Model file for the job. Use its own axes, mm. A direction names the side the tool comes from. Round coordinates to 2 decimals unless told otherwise and drop trailing zeros. Loops run counter-clockwise (first coordinate to the right, second up) from the corner with the lowest first, then second, coordinate; pieces in that order, holes last. Notation, with made-up numbers: (48.5, 26) - (93.5, 26) arc R27 cw to (93.5, 51) - close; hole circle Ø6 at (86, -24.5). An arc over 180 degrees is marked (long way). Use one line per item in the form item = value.
from build123d import *

# Parameters (mm, degrees)
SKETCH2_W           = 60
SKETCH2_H           = 110
BOSS_EXTRUDE1_DEPTH = 1.5748
BOSS_EXTRUDE2_DEPTH = 6
BOSS_EXTRUDE3_DEPTH = 6
SKETCH6_W           = 6
SKETCH6_H           = 12.6
SKETCH6_W_2         = 7.6
SKETCH6_H_2         = 9.9
SKETCH6_W_3         = 3
SKETCH6_H_3         = 4.5
SKETCH6_W_4         = 16.25
SKETCH6_H_4         = 13.5
SKETCH6_W_5         = 3.65
SKETCH6_H_5         = 4.8
BOSS_EXTRUDE4_DEPTH = 1
SKETCH7_R           = 1.375
SKETCH7_R_2         = 1.625
CUT_EXTRUDE1_DEPTH  = 126.443214245
SKETCH8_R           = 0.9
BOSS_EXTRUDE5_DEPTH = 1
SKETCH9_W           = 2.7
SKETCH9_H           = 1.5
BOSS_EXTRUDE6_DEPTH = 1
CUT_EXTRUDE2_DEPTH  = 3


with BuildPart() as part:
    # Sketch2 → Boss-Extrude1 (new body)
    with BuildSketch(Plane(origin=(0, 0, 0), x_dir=(1, 0, 0), z_dir=(0, 1, 0))):
        with Locations((30, 55)):
            Rectangle(SKETCH2_W, SKETCH2_H)
    extrude(amount=-BOSS_EXTRUDE1_DEPTH)

    # Sketch3 → Boss-Extrude2 (add)
    with BuildSketch(Plane(origin=(0, 0, 0), x_dir=(1, 0, 0), z_dir=(0, 1, 0))):
        Polygon((0.6425, 8.49), (6.3575, 8.49), (6.3575, 21.5075), (7.31, 21.5075), (7.31, 28.4925), (6.3575, 28.4925), (6.3575, 41.51), (0.6425, 41.51), align=None)
    extrude(amount=BOSS_EXTRUDE2_DEPTH)

    # Sketch5 → Boss-Extrude3 (add)
    with BuildSketch(Plane(origin=(0, 0, 0), x_dir=(1, 0, 0), z_dir=(0, 1, 0))):
        Polygon((49.05, 109.3575), (10.95, 109.3575), (10.95, 103.6425), (26.5075, 103.6425), (26.5075, 102.69), (33.4925, 102.69), (33.4925, 103.6425), (49.05, 103.6425), align=None)
    extrude(amount=BOSS_EXTRUDE3_DEPTH)

    # Sketch6 → Boss-Extrude4 (add)
    with BuildSketch(Plane(origin=(0, 0, 0), x_dir=(1, 0, 0), z_dir=(0, 1, 0))):
        with Locations((33, 67)):
            Rectangle(SKETCH6_W, SKETCH6_H)
        Polygon((30.875, 33.85), (30.875, 27.65), (30.6, 27.375), (24.4, 27.375), (24.125, 27.65), (24.125, 33.85), (24.4, 34.125), (30.6, 34.125), align=None)
        with Locations((18.25, 13)):
            Rectangle(SKETCH6_W_2, SKETCH6_H_2)
        with Locations((23.5, 3.25)):
            Rectangle(SKETCH6_W_3, SKETCH6_H_3)
        with Locations((50.625, 17.25)):
            Rectangle(SKETCH6_W_4, SKETCH6_H_4)
        with Locations((57.75, 38)):
            Rectangle(SKETCH6_W_5, SKETCH6_H_5)
        with Locations((57.75, 45.25)):
            Rectangle(SKETCH6_W_5, SKETCH6_H_5)
        with Locations((51, 45)):
            Rectangle(SKETCH6_W_5, SKETCH6_H_5)
        with Locations((51, 35.5)):
            Rectangle(SKETCH6_W_5, SKETCH6_H_5)
    extrude(amount=BOSS_EXTRUDE4_DEPTH)

    # Sketch7 → Cut-Extrude1 (cut, through all)
    with BuildSketch(Plane(origin=(0, 0, 0), x_dir=(1, 0, 0), z_dir=(0, 1, 0))):
        with Locations(Location((3.75, 52, 0), (0, 0, 270))):
            Circle(SKETCH7_R)
        with Locations(Location((3.75, 70.5, 0), (0, 0, 270))):
            Circle(SKETCH7_R)
        with Locations(Location((3.75, 79.5, 0), (0, 0, 270))):
            Circle(SKETCH7_R)
        with Locations(Location((3.75, 88.5, 0), (0, 0, 270))):
            Circle(SKETCH7_R)
        with Locations(Location((3.75, 97.5, 0), (0, 0, 270))):
            Circle(SKETCH7_R)
        with Locations(Location((3.75, 61, 0), (0, 0, 270))):
            Circle(SKETCH7_R)
        with Locations(Location((5, 106, 0), (0, 0, 270))):
            Circle(SKETCH7_R_2)
        with Locations(Location((55, 106, 0), (0, 0, 270))):
            Circle(SKETCH7_R_2)
        with Locations(Location((55, 4, 0), (0, 0, 270))):
            Circle(SKETCH7_R_2)
        with Locations(Location((5, 4, 0), (0, 0, 270))):
            Circle(SKETCH7_R_2)
    extrude(amount=-CUT_EXTRUDE1_DEPTH, mode=Mode.SUBTRACT)

    # Sketch8 → Boss-Extrude5 (add)
    with BuildSketch(Plane(origin=(0, 1, 0), x_dir=(1, 0, 0), z_dir=(0, 1, 0))):
        with Locations(Location((57.75, 38, 0), (0, 0, 270))):
            Circle(SKETCH8_R)
        with Locations(Location((57.75, 45.25, 0), (0, 0, 270))):
            Circle(SKETCH8_R)
        with Locations(Location((51, 45, 0), (0, 0, 270))):
            Circle(SKETCH8_R)
        with Locations(Location((51, 35.5, 0), (0, 0, 270))):
            Circle(SKETCH8_R)
    extrude(amount=BOSS_EXTRUDE5_DEPTH)

    # Sketch9 → Boss-Extrude6 (add)
    with BuildSketch(Plane(origin=(0, 0, 0), x_dir=(1, 0, 0), z_dir=(0, 1, 0))):
        with Locations((57.5, 50)):
            Rectangle(SKETCH9_W, SKETCH9_H)
        with Locations((57.5, 54.25)):
            Rectangle(SKETCH9_W, SKETCH9_H)
        with Locations((57.5, 58.75)):
            Rectangle(SKETCH9_W, SKETCH9_H)
        with Locations((57.5, 63.25)):
            Rectangle(SKETCH9_W, SKETCH9_H)
        with Locations((57.5, 67.75)):
            Rectangle(SKETCH9_W, SKETCH9_H)
        with Locations((57.5, 72.25)):
            Rectangle(SKETCH9_W, SKETCH9_H)
        with Locations((57.5, 76.75)):
            Rectangle(SKETCH9_W, SKETCH9_H)
        with Locations((57.5, 81.25)):
            Rectangle(SKETCH9_W, SKETCH9_H)
        with Locations((57.5, 85.75)):
            Rectangle(SKETCH9_W, SKETCH9_H)
        with Locations((57.5, 90.25)):
            Rectangle(SKETCH9_W, SKETCH9_H)
        with Locations((57.5, 94.75)):
            Rectangle(SKETCH9_W, SKETCH9_H)
        with Locations((57.5, 99.25)):
            Rectangle(SKETCH9_W, SKETCH9_H)
    extrude(amount=BOSS_EXTRUDE6_DEPTH)

    # Sketch10 → Cut-Extrude2 (cut)
    with BuildSketch(Plane(origin=(0, 6, 0), x_dir=(1, 0, 0), z_dir=(0, 1, 0))):
        Polygon((1.3925, 40.76), (1.3925, 9.24), (5.6075, 9.24), (5.6075, 22.2575), (6.56, 22.2575), (6.56, 27.7425), (5.6075, 27.7425), (5.6075, 40.76), align=None)
        Polygon((32.7425, 104.3925), (48.3, 104.3925), (48.3, 108.6075), (11.7, 108.6075), (11.7, 104.3925), (27.2575, 104.3925), (27.2575, 103.44), (32.7425, 103.44), align=None)
    extrude(amount=-CUT_EXTRUDE2_DEPTH, mode=Mode.SUBTRACT)


solid = part.part
1. Pull direction Z, two halves, no side cores. Call faces 1 (the flat face through (1, 6, -25)), 2 (the flat face through (30, 3, -109.358)), 3 (the flat face through (40, 5, -104.392)): +Z half, -Z half, draft (parallel to the pull), parting line (faces both ways), or undercut.
Geometry check:
face_1 = draft
face_2 = -Z half
face_3 = undercut
2. Wall check: probe 1 along X at (y, z) = (-0.5, -4) (3 decimals); probe 2 along X at (y, z) = (-1.05, -70.5) (3 decimals); probe 3 along Z at (x, y) = (3, 3.5). Give the ranges that are in metal, low to high.
Geometry check:
probe_1 = 0 to 3.375, 6.625 to 53.375, 56.625 to 60
probe_2 = 0 to 2.375, 5.125 to 60
probe_3 = -41.51 to -40.76, -9.24 to -8.49
3. Cut at C-C, the plane x = 15.5. Give the cut face in (y, z), plus the area to 3 significant figures.
Geometry check:
outline = (-1.57, -110) - (0, -110) - (0, -109.36) - (6, -109.36) - (6, -108.61) - (3, -108.61) - (3, -104.39) - (6, -104.39) - (6, -103.64) - (0, -103.64) - (0, -17.95) - (1, -17.95) - (1, -8.05) - (0, -8.05) - (0, 0) - (-1.57, 0) - close
area = 205 mm^2
4. Cut at A-A, the plane y = 4.5. Give the number of separate pieces and of enclosed holes in the cut face, plus the area to 3 significant figures.
Geometry check:
separate_pieces = 2
enclosed_holes = 2
area = 122 mm^2
5. Flat gauge pins, fed straight in: pin 1 (6 mm diameter, centred on x = 15, z = -75, fed in from +Y); pin 2 (0.8 mm diameter, centred on x = 57.5, z = -58.5, fed in from +Y); pin 3 (1 mm diameter, centred on x = 20, y = 2.5, fed in from -Z). Where does each tip first touch, or does it go through?
Geometry check:
pin_1 = 0
pin_2 = 1
pin_3 = -109.36
6. Tool access for faces 4 (the flat face through (5.608, 5, -34)), 5 (the flat face through (30, 3, -102.69)), 6 (the flat face through (41, 3, -103.642)): list every direction of +Z, -Z, +X, -X, +Y, -Y with a clear straight run to the whole face (end or side of a thin tool).
Geometry check:
face_4 = +Y
face_5 = +X, -X, +Y
face_6 = +X, +Y
7. Cut at B-B, the plane z = -31.5. Give the cut face in (x, y) (1 decimal), plus the area to 3 significant figures.
Geometry check:
outline = (0, -1.6) - (60, -1.6) - (60, 0) - (30.9, 0) - (30.9, 1) - (24.1, 1) - (24.1, 0) - (6.4, 0) - (6.4, 6) - (5.6, 6) - (5.6, 3) - (1.4, 3) - (1.4, 6) - (0.6, 6) - (0.6, 0) - (0, 0) - close
area = 123 mm^2
8. Cut at D-D, the plane x = 41. Give the cut face in (y, z), plus the area to 3 significant figures.
Geometry check:
outline = (-1.57, -110) - (0, -110) - (0, -109.36) - (6, -109.36) - (6, -108.61) - (3, -108.61) - (3, -104.39) - (6, -104.39) - (6, -103.64) - (0, -103.64) - (0, 0) - (-1.57, 0) - close
area = 195 mm^2
